from build123d import *

# Parameters (mm, degrees)
SKETCH1_W               = 80
SKETCH1_H               = 45.4
SKETCH1_R               = 1.65
BOSS_EXTRUDE1_DEPTH     = 12.5
SKETCH2_W               = 5
SKETCH2_H               = 45.4
BOSS_EXTRUDE2_DEPTH     = 10.5
CUT_EXTRUDE1_DEPTH      = 7.8
CUT_EXTRUDE1_DEPTH_BACK = 93.830005925
SKETCH3_W               = 80
SKETCH3_H               = 12.2
SKETCH4_W               = 30
SKETCH4_H               = 8
BOSS_EXTRUDE3_DEPTH     = 44.2
SKETCH5_R               = 12
CUT_EXTRUDE2_DEPTH      = 45
CUT_EXTRUDE3_DEPTH      = 96.828388278
CUT_EXTRUDE3_DEPTH_BACK = 96.828388278
SKETCH6_R               = 2.6
FILLET1_SIZE            = 6
FILLET1_SIZE_2          = 15
SKETCH8_R               = 3.5
CUT_EXTRUDE5_DEPTH      = 10.5
SKETCH12_W              = 45
SKETCH12_H              = 12.25
CUT_EXTRUDE8_DEPTH      = 10.5
SKETCH13_W              = 14
SKETCH13_H              = 23.274164218
CUT_EXTRUDE10_DEPTH     = 10
SKETCH15_R              = 2.75
BOSS_EXTRUDE6_DEPTH     = 2
SKETCH16_W              = 43.029059925
SKETCH16_H              = 12.5
CUT_EXTRUDE11_DEPTH     = 12.5
CHAMFER2_SIZE2          = 12.5
CHAMFER2_SIZE           = 4.549627928
SKETCH17_R              = 2.2
CUT_EXTRUDE12_DEPTH     = 10
CUT_EXTRUDE13_DEPTH     = 102.559280367
SKETCH19_W              = 5
SKETCH19_H              = 24.2
BOSS_EXTRUDE7_DEPTH     = 5
SKETCH20_W              = 1
SKETCH20_H              = 12.2
CUT_EXTRUDE14_DEPTH     = 102.559280367
SKETCH21_W              = 5
SKETCH21_H              = 9.5
BOSS_EXTRUDE8_DEPTH     = 12.2
FILLET2_R               = 1
FILLET3_R               = 13
CHAMFER1_SIZE           = 2
SKETCH22_W              = 38.479431997
SKETCH22_H              = 1
BOSS_EXTRUDE9_DEPTH     = 3
SKETCH23_W              = 38.4
SKETCH23_H              = 1
BOSS_EXTRUDE10_DEPTH    = 3
CHAMFER3_SIZE           = 3


# Some blends are built 0.0001 mm under size
with BuildPart() as part:
    # Sketch1 → Boss-Extrude1 (new body)
    with BuildSketch(Plane.XY):
        with Locations((40, 22.7)):
            Rectangle(SKETCH1_W, SKETCH1_H)
        with Locations((8.499989197, 32.7)):
            Circle(SKETCH1_R, mode=Mode.SUBTRACT)
        with Locations((28.499989197, 32.7)):
            Circle(SKETCH1_R, mode=Mode.SUBTRACT)
        with Locations((28.499989197, 12.7)):
            Circle(SKETCH1_R, mode=Mode.SUBTRACT)
        with Locations((8.499989197, 12.7)):
            Circle(SKETCH1_R, mode=Mode.SUBTRACT)
    extrude(amount=BOSS_EXTRUDE1_DEPTH)

    # Sketch2 → Boss-Extrude2 (add)
    with BuildSketch(Plane(origin=(0, 0, 0), x_dir=(-1, 0, 0), z_dir=(0, 0, -1))):
        with Locations((-2.5, 22.7)):
            Rectangle(SKETCH2_W, SKETCH2_H)
    extrude(amount=BOSS_EXTRUDE2_DEPTH)

    # Sketch3 → Cut-Extrude1 (cut, two sides: drawn at the far end of the back side and taken through both)
    with BuildSketch(Plane.XY.offset(-CUT_EXTRUDE1_DEPTH_BACK)):
        with Locations((40, 22.7)):
            Rectangle(SKETCH3_W, SKETCH3_H)
    extrude(amount=CUT_EXTRUDE1_DEPTH + CUT_EXTRUDE1_DEPTH_BACK, mode=Mode.SUBTRACT)

    # Sketch4 → Boss-Extrude3 (add)
    with BuildSketch(Plane(origin=(0, 0, 0), x_dir=(-1, 0, 0), z_dir=(0, 0, -1))):
        with Locations((-54.5, 4)):
            Rectangle(SKETCH4_W, SKETCH4_H)
    extrude(amount=BOSS_EXTRUDE3_DEPTH)

    # Sketch5 → Cut-Extrude2 (cut)
    with BuildSketch(Plane(origin=(0, 8, 0), x_dir=(1, 0, 0), z_dir=(0, 1, 0))):
        with Locations(Location((54.495569327, 23.5, 0), (0, 0, 270))):
            Circle(SKETCH5_R)
    extrude(amount=-CUT_EXTRUDE2_DEPTH, mode=Mode.SUBTRACT)

    # Sketch6 → Cut-Extrude3 (cut, two sides: drawn at the far end of the back side and taken through both)
    with BuildSketch(Plane.XZ.offset(-16.6).offset(-CUT_EXTRUDE3_DEPTH_BACK)):
        with Locations((54.495569327, -39.201340104)):
            Circle(SKETCH6_R)
        with Locations((65.809277826, -34.515048603)):
            Circle(SKETCH6_R)
        with Locations((43.181860828, -34.515048603)):
            Circle(SKETCH6_R)
        with Locations((43.181860828, -11.887631605)):
            Circle(SKETCH6_R)
        with Locations((65.809277826, -11.887631605)):
            Circle(SKETCH6_R)
    extrude(amount=CUT_EXTRUDE3_DEPTH + CUT_EXTRUDE3_DEPTH_BACK, mode=Mode.SUBTRACT)

    # Fillet1
    # a fillet whose section is not a circle: 15, 6 mm, written as the material it takes off along each edge
    with BuildSketch(Plane(origin=(39.5, -37.5, -44.2), x_dir=(0, 0, 1), z_dir=(0, 1, 0)), Plane(origin=(69.5, 45.5, -44.2), x_dir=(0, 0, 1), z_dir=(0, -1, 0))) as fillet1_piece_1:
        with BuildLine():
            Bezier((FILLET1_SIZE, 0), (0, 0), (0, FILLET1_SIZE_2), weights=[1, 0.428571429, 1])
            Line((0, FILLET1_SIZE_2), (0, 0))
            Line((0, 0), (FILLET1_SIZE, 0))
        make_face()
    extrude(amount=83, mode=Mode.SUBTRACT)

    # Sketch8 → Cut-Extrude5 (cut)
    with BuildSketch(Plane.XY.offset(12.5)):
        with Locations((8.499989197, 32.7)):
            Circle(SKETCH8_R)
        with Locations((28.499989197, 32.7)):
            Circle(SKETCH8_R)
        with Locations((8.499989197, 12.7)):
            Circle(SKETCH8_R)
        with Locations((28.499989197, 12.7)):
            Circle(SKETCH8_R)
    extrude(amount=-CUT_EXTRUDE5_DEPTH, mode=Mode.SUBTRACT)

    # Sketch12 → Cut-Extrude8 (cut)
    with BuildSketch(Plane.XY.offset(12.5)):
        with Locations((22.5, 39.275)):
            Rectangle(SKETCH12_W, SKETCH12_H)
    extrude(amount=-CUT_EXTRUDE8_DEPTH, mode=Mode.SUBTRACT)

    # Sketch13 → Cut-Extrude10 (cut)
    with BuildSketch(Plane(origin=(0, 8, 0), x_dir=(1, 0, 0), z_dir=(0, 1, 0))):
        with Locations((54.495569327, 39.201340104)):
            Rectangle(SKETCH13_W, SKETCH13_H)
    extrude(amount=-CUT_EXTRUDE10_DEPTH, mode=Mode.SUBTRACT)

    # Sketch15 → Boss-Extrude6 (add)
    with BuildSketch(Plane(origin=(0, 8, 0), x_dir=(1, 0, 0), z_dir=(0, 1, 0))):
        with Locations(Location((54.495569327, 7.201340104, 0), (0, 0, 90))):
            Circle(SKETCH15_R)
    extrude(amount=BOSS_EXTRUDE6_DEPTH)

    # Sketch16 → Cut-Extrude11 (cut)
    with BuildSketch(Plane(origin=(0, 45.4, 0), x_dir=(1, 0, 0), z_dir=(0, 1, 0))):
        with Locations((53.485470038, -6.25)):
            Rectangle(SKETCH16_W, SKETCH16_H)
    extrude(amount=-CUT_EXTRUDE11_DEPTH, mode=Mode.SUBTRACT)

    # Chamfer2
    chamfer2_edges = [part.edges().sort_by_distance(p)[0] for p in [
        (75, 32.9, 6.25),
    ]]
    chamfer2_side = [part.faces().sort_by_distance(p)[0] for p in [
        (74.909007441, 32.9, 6.25),
    ]]
    chamfer(chamfer2_edges, length=CHAMFER2_SIZE - 0.0001, length2=CHAMFER2_SIZE2 - 0.0001, reference=chamfer2_side[0])  # a hair under: the kernel refuses the full size

    # Sketch17 → Cut-Extrude12 (cut)
    with BuildSketch(Plane(origin=(80, 0, 0), x_dir=(0, 0, -1), z_dir=(1, 0, 0))):
        with Locations((-7.3, 39.15)):
            Circle(SKETCH17_R)
    extrude(amount=-CUT_EXTRUDE12_DEPTH, mode=Mode.SUBTRACT)

    # Sketch18 → Cut-Extrude13 (cut, through all)
    with BuildSketch(Plane(origin=(80, 0, 0), x_dir=(0, 0, -1), z_dir=(1, 0, 0))):
        Polygon((-7.8, 28.8), (-6.8, 28.8), (-7.8, 29.3), align=None)
        Polygon((-7.8, 16.6), (-7.8, 16.1), (-6.8, 16.6), align=None)
    extrude(amount=-CUT_EXTRUDE13_DEPTH, mode=Mode.SUBTRACT)

    # Sketch19 → Boss-Extrude7 (add)
    with BuildSketch(Plane(origin=(0, 0, 0), x_dir=(-1, 0, 0), z_dir=(0, 0, -1))):
        with Locations((-77.5, 22.7)):
            Rectangle(SKETCH19_W, SKETCH19_H)
    extrude(amount=BOSS_EXTRUDE7_DEPTH)

    # Sketch20 → Cut-Extrude14 (cut, through all)
    with BuildSketch(Plane(origin=(80, 0, 0), x_dir=(0, 0, -1), z_dir=(1, 0, 0))):
        with Locations((0.5, 22.7)):
            Rectangle(SKETCH20_W, SKETCH20_H)
    extrude(amount=-CUT_EXTRUDE14_DEPTH, mode=Mode.SUBTRACT)

    # Sketch21 → Boss-Extrude8 (add)
    with BuildSketch(Plane(origin=(0, 16.6, 0), x_dir=(1, 0, 0), z_dir=(0, 1, 0))):
        with Locations((2.5, 5.75)):
            Rectangle(SKETCH21_W, SKETCH21_H)
    extrude(amount=BOSS_EXTRUDE8_DEPTH)

    # Fillet2
    fillet2_edges = [part.edges().sort_by_distance(p)[0] for p in [
        (77.5, 16.6, -1),
        (77.5, 28.8, -1),
        (2.5, 16.6, -1),
        (2.5, 28.8, -1),
    ]]
    fillet(fillet2_edges, radius=FILLET2_R)

    # Fillet3
    # the kernel refuses this fillet: 13 mm, written as the material it adds along each edge
    with BuildSketch(Plane(origin=(80, 10.6, 0), x_dir=(0, -1, 0), z_dir=(-1, 0, 0)), Plane(origin=(75, 34.8, 0), x_dir=(0, 1, 0), z_dir=(1, 0, 0))) as fillet3_piece_1:
        with BuildLine():
            CenterArc((10.246950766, -13), FILLET3_R, 90, 52.020127555)
            Line((0, -5), (0, 0))
            Line((0, 0), (10.246950766, 0))
        make_face()
    extrude(amount=5)

    # Chamfer1
    chamfer1_edges = [part.edges().sort_by_distance(p)[0] for p in [
        (54.495569327, 10, -4.451340104),
    ]]
    chamfer(chamfer1_edges, length=CHAMFER1_SIZE - 0.0001)  # a hair under: the kernel refuses the full size

    # Sketch22 → Boss-Extrude9 (add)
    with BuildSketch(Plane.XY.offset(12.5)):
        with Locations((51.210656074, 32.4)):
            Rectangle(SKETCH22_W, SKETCH22_H)
    extrude(amount=BOSS_EXTRUDE9_DEPTH)

    # Sketch23 → Boss-Extrude10 (add)
    with BuildSketch(Plane(origin=(0, 0, 0), x_dir=(-1, 0, 0), z_dir=(0, 0, -1))):
        with Locations((-51.250372072, 32.4)):
            Rectangle(SKETCH23_W, SKETCH23_H)
    extrude(amount=BOSS_EXTRUDE10_DEPTH)

    # Chamfer3
    chamfer3_edges = [part.edges().sort_by_distance(p)[0] for p in [
        (51.210656074, 31.9, 12.5),
        (51.250372072, 31.9, 0),
    ]]
    chamfer(chamfer3_edges, length=CHAMFER3_SIZE - 0.0001)  # a hair under: the kernel refuses the full size


solid = part.part
Read the model definition and answer for the solid it produces. Units are mm, in the model's axes. A direction names the side the tool comes from. Coordinates: 2 decimals unless noted, no trailing zeros. Order: outer loops, then holes, each group sorted by start corner. A loop starts at its lowest first (then second) coordinate and runs counter-clockwise, first axis right, second up. Notation, with made-up numbers: M -18.5,41.25 L 17.5,41.25 A6 ccw 17.5,45.25 Z; hole C 75,31.5 d2. An arc over 180 degrees is marked long. Put each result on its own line as item: value. Start each with the question number.
Item 1: For faces 4 (the face through (78, 23, -1)), 5 (the face through (61.496, 4, -38)), 6 (the face through (51.5, 30.4, -1.5)), determine the directions among +Z, -Z, +X, -X, +Y, -Y from which every point of the face is accessible in a straight line to the end or side of a thin tool.
Item 2: Consider probe 1 along X at (y, z) = (33, 6); probe 2 along Y at (x, z) = (44, 5); probe 3 along X at (y, z) = (33, -7). Determine where each line is inside the solid, lowest interval first. Write a range as [from, to].
Item 3: Section D-D, the plane y = 12.7 is taken. Determine the outline of the cut face in (x, z).
Item 4: Given pin 1 Ø15 at (x, z) = (55.5, 9.5) entering from +Y; pin 2 Ø12 at (x, y) = (64.5, 40.5) entering from -Z; pin 3 Ø6 at (x, z) = (43.18, -11.89) entering from +Y; pin 4 Ø5.5 at (x, y) = (8.5, 32.7) entering from -Z, each flat-ended and moving along its own axis, determine where each tip first touches the part or whether it passes through.
Item 5: Section C-C, the plane x = 20.5 is taken. Determine the outline of the cut face in (y, z).
Item 6: The mould has two halves that part along Y. Classify faces 1 (the face through (9, 45.4, 0.4)), 2 (the face through (69.5, 4, -19)), 3 (the face through (41, 28.8, 3)): +Y half, -Y half, draft (parallel to the pull), parting line (faces both ways), or undercut.
Item 7: Section A-A, the plane y = 26 is taken. Determine the outline of the cut face in (x, z).
Item 8: Section B-B, the plane z = -25.5 is taken. Determine the outline of the cut face in (x, y).
Computed:
1. face 4: +X, -X
1. face 5: -Z, +Y, -Y
1. face 6: -Z
2. probe 1: x = [0, 5.01], [11.99, 25.01], [70.49, 80]
2. probe 2: y = [0, 16.6], [28.8, 32.9]
2. probe 3: x = [0, 5]
3. outline: M 0,-10.5 L 5,-10.5 L 5,0 L 6.85,0 L 6.85,2 L 5,2 L 5,12.5 L 0,12.5 Z; M 10.15,0 L 26.85,0 L 26.85,2 L 25,2 L 25,12.5 L 12,12.5 L 12,2 L 10.15,2 Z; M 30.15,0 L 75,0 L 75,-5 L 80,-5 L 80,12.5 L 32,12.5 L 32,2 L 30.15,2 Z
4. pin 1: stops at y = 32.9
4. pin 2: passes through
4. pin 3: stops at y = 8
4. pin 4: stops at z = 0
5. outline: M 0,0 L 16.6,0 L 16.6,6.8 L 16.1,7.8 L 29.3,7.8 L 28.8,6.8 L 28.8,0 L 45.4,0 L 45.4,2 L 33.15,2 L 33.15,12.5 L 0,12.5 Z
6. face 1: +Y half
6. face 2: draft
6. face 3: undercut
7. outline: M 0,-10.5 L 5,-10.5 L 5,-1 L 0,-1 Z; M 0,7.8 L 80,7.8 L 80,12.5 L 0,12.5 Z; M 75,-5 L 80,-5 L 80,-1 L 75,-1 Z
8. outline: M 39.5,0 L 42.66,0 L 42.66,8 L 39.5,8 Z; M 66.33,0 L 69.5,0 L 69.5,8 L 66.33,8 Z
